Read the model definition and answer for the solid it produces. Units are mm, in the model's axes. Coordinates: 2 decimals unless noted, no trailing zeros. Order: outer loops, then holes, each group sorted by start corner. A loop starts at its lowest first (then second) coordinate and runs counter-clockwise, first axis right, second up. Notation, with made-up numbers: M 8.25,63.25 L 35.25,63.25 A23 cw 35.25,92.25 Z; hole C -1,34.25 d10. An arc over 180 degrees is marked long. Use a Markdown table: item, result. Add a question column.
1) Each of these flat-tipped pins is pushed along its axis until it touches: pin 1 Ø1.5 at (y, z) = (-2, 6) entering from -X; pin 2 Ø3 at (y, z) = (-5, 25.5) entering from -X; pin 3 Ø4 at (x, z) = (-10, 11.5) entering from -Y; pin 4 Ø3 at (x, y) = (-3, -4) entering from +Z. Where does it stop, or does it pass through?
2) Find section A-A on y = -0.75. Write down the section's boundary in (x, z), plus the area to 3 significant figures.
3) Find section C-C on x = 3. Write down the section's boundary in (y, z).
4) Find the intervals of material crossed by probe 1 along X at (y, z) = (-3.5, 27.5); probe 2 along X at (y, z) = (-5.25, 32); probe 3 along Z at (x, y) = (-9, -5.25), in increasing order. Write a range as [from, to].
5) Find section B-B on z = 39. Write down the section's boundary in (x, y).
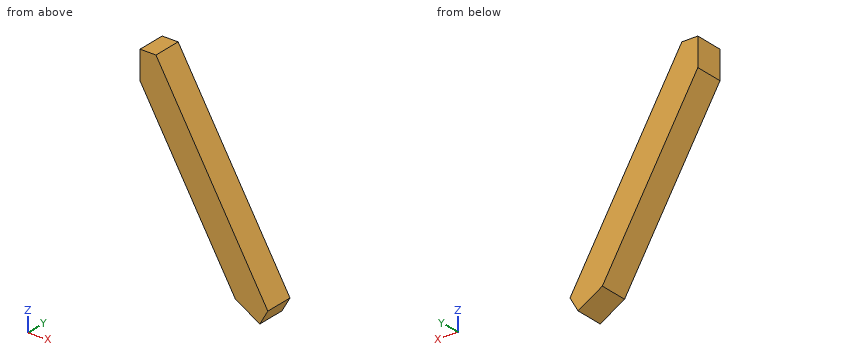
from build123d import *

# Parameters (mm, degrees)
F1_DEPTH = 6.6


with BuildPart() as f1:
    # F0 (on Front) → F1 (new body)
    with BuildSketch(Plane.XZ):
        Polygon((-20.828086, 43.877387), (-24.60951, 37.198508), (-1.976367, -1.251827), (5.698425, -1.187197), align=None)
        Polygon((-24.60951, 43.845072), (-24.60951, 37.198508), (-20.828086, 43.877387), align=None)
        Polygon((5.698425, -1.187197), (-1.976367, -1.251827), (3.807712, -4.526636), align=None)
    extrude(amount=F1_DEPTH)


solid = f1.part
Check result:
| question | item | result |
|---|---|---|
| 1 | pin 1 | stops at x = -6.69 |
| 1 | pin 2 | stops at x = -18.61 |
| 1 | pin 3 | stops at y = -6.6 |
| 1 | pin 4 | stops at z = 16.14 |
| 2 | outline | M -24.61,37.2 L -1.98,-1.25 L 3.81,-4.53 L 5.7,-1.19 L -20.83,43.88 L -24.61,43.85 Z |
| 2 | area | 347 mm2 |
| 3 | outline | M -6.6,-4.07 L 0,-4.07 L 0,3.4 L -6.6,3.4 Z |
| 4 | probe 1 | x = [-18.9, -11.19] |
| 4 | probe 2 | x = [-21.55, -13.84] |
| 4 | probe 3 | z = [10.68, 23.78] |
| 5 | outline | M -24.61,-6.6 L -17.96,-6.6 L -17.96,0 L -24.61,0 Z |
